Geometry: final body of the model. Coordinates: model frame, mm. Face numbers are marked on the shaded views. A direction names the side the tool comes from. Coordinates: 2 decimals unless noted, no trailing zeros. Order: outer loops, then holes, each group sorted by start corner. A loop starts at its lowest first (then second) coordinate and runs counter-clockwise, first axis right, second up. Notation, with made-up numbers: M -13,11.5 L 24,11.5 A28 ccw 24,43.5 Z; hole C 5,12.5 d1. An arc over 180 degrees is marked long. Use CSV: the item, a comma, the result in double quotes. Start each with the question number.
1. Section query D-D on z = 14.5. Return the cut outline in (x, y).
2. Section query A-A on z = 4.5. Return the cut outline in (x, y).
3. Material intervals for line 1 (X direction, y = 1, z = 3); line 2 (Y direction, x = -1.5, z = 8); line 3 (Y direction, x = 0, z = 16), sorted ascending.
4. Pull-direction query (X, two-part tool) for the marked faces 1, 2 and 3; classes: pulls with the +X half, pulls with the -X half, needs draft (parallel to the pull), parting line crosses it, or undercut.
5. Section query B-B on y = 0. Return the cut outline in (x, z).
6. First-contact query: P1, Ø6, axis at y = -2.5, z = 22, coming from the -X side; P2, Ø4, axis at y = -12, z = 9, coming from the -X side; P3, Ø12, axis at y = 12.5, z = 10.5, coming from the +X side. Flat tips, straight axial feed; report the tip coordinate or a pass-through.
7. Section query C-C on x = 0. Return the cut outline in (y, z), and give its area (3 significant figures).
8. Set-up query: the marked faces 4 and 5. Return all of +Z, -Z, +X, -X, +Y, -Y with unobstructed straight access to the full face (end or side cutting, diameter ignored); none if empty.
from build123d import *

# Parameters (mm, degrees)
F0_W     = 50.8
F0_H     = 38.1
F1_DEPTH = 25.4
F1_TAPER = 5
F2_R     = 8.89
F3_DEPTH = 12.7
F4_R     = 5.08
F5_DEPTH = 38.101
F6_T     = -2.54


with BuildPart() as f1:
    # F0 (on Top) → F1 (new body)
    with BuildSketch(Plane.XY):
        Rectangle(F0_W, F0_H)
    extrude(amount=F1_DEPTH, taper=F1_TAPER)

    # F2 (on face) → F3 (join)
    with BuildSketch(Plane.XY.offset(25.4)):
        Circle(F2_R)
    extrude(amount=F3_DEPTH)

    # F4 (on face) → F5 (cut, through all)
    with BuildSketch(Plane.XY.offset(38.1)):
        Circle(F4_R)
    extrude(amount=-F5_DEPTH, mode=Mode.SUBTRACT)

    # F6
    f6_openings = [f1.faces().sort_by_distance(p)[0] for p in [
        (24.765, 0, 0),
    ]]
    offset(amount=F6_T, openings=f6_openings, kind=Kind.INTERSECTION)


solid = f1.part
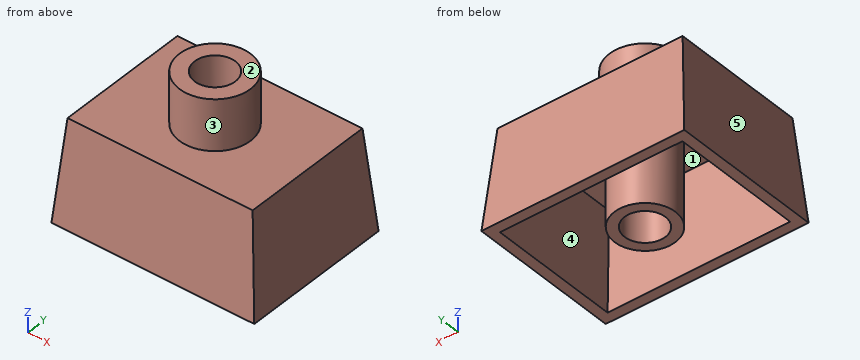
Results list:
1,outline,"M -24.13,-17.78 L 24.13,-17.78 L 24.13,17.78 L -24.13,17.78 Z; C 0,0 d15.24; hole M -21.58,-15.23 L 21.58,-15.23 L 21.58,15.23 L -21.58,15.23 Z; hole C 0,0 d10.16"
2,outline,"M -25.01,-18.66 L 25.01,-18.66 L 25.01,18.66 L -25.01,18.66 Z; C 0,0 d15.24; hole M -22.46,-16.11 L 22.46,-16.11 L 22.46,16.11 L -22.46,16.11 Z; hole C 0,0 d10.16"
3,line 1,"x = -25.14 to -22.59, -7.55 to -4.98, 4.98 to 7.55, 22.59 to 25.14"
3,line 2,"y = -18.35 to -15.8, -7.47 to -4.85, 4.85 to 7.47, 15.8 to 18.35"
3,line 3,"y = -17.65 to -15.1, -7.62 to -5.08, 5.08 to 7.62, 15.1 to 17.65"
4,face 1,"undercut"
4,face 2,"needs draft"
4,face 3,"parting line crosses it"
5,outline,"M -25.4,0 L -22.85,0 L -20.85,22.86 L -7.62,22.86 L -7.62,0 L -5.08,0 L -5.08,38.1 L -8.89,38.1 L -8.89,25.4 L -23.18,25.4 Z; M 5.08,0 L 7.62,0 L 7.62,22.86 L 20.85,22.86 L 22.85,0 L 25.4,0 L 23.18,25.4 L 8.89,25.4 L 8.89,38.1 L 5.08,38.1 Z"
6,P1,"stops at x = -23.74"
6,P2,"stops at x = -24.79"
6,P3,"stops at x = 25.01"
7,outline,"M -19.05,0 L -16.5,0 L -14.5,22.86 L -7.62,22.86 L -7.62,0 L -5.08,0 L -5.08,38.1 L -8.89,38.1 L -8.89,25.4 L -16.83,25.4 Z; M 5.08,0 L 7.62,0 L 7.62,22.86 L 14.5,22.86 L 16.5,0 L 19.05,0 L 16.83,25.4 L 8.89,25.4 L 8.89,38.1 L 5.08,38.1 Z"
7,area,"390 mm²"
8,face 4,"-Z"
8,face 5,"+Z, -X, +Y, -Y"
